Source: three-view drawing plus pictorial views. Frame: mm from the lowest corner of the part. Coordinates: 2 decimals unless noted, no trailing zeros. Write each loop counter-clockwise with the first axis right and the second up, starting at its lowest first coordinate (ties: lowest second). Pieces come first, ordered by that corner, then holes. Notation, with made-up numbers: M -28.75,16 L 15.25,16 A16 cw 15.25,38 Z; hole C 35.5,80 d11. An arc over 180 degrees is marked long. Write item = value, one per line. Start each with the question number.
Item 1: Section A-A on y = 1.2. Output: boundary loops of the cut face in (x, z) (1 decimal).
Item 2: Ray query, L1, parallel to X at y = 1, z = 15.5. Return the intervals inside material, ascending. Write a range as [from, to].
Item 3: Section B-B on z = 36.5. Output: boundary loops of the cut face in (x, y).
Item 4: First-contact query: pin 1 Ø1.6 at (y, z) = (2.5, 42.5) entering from -X; pin 2 Ø3 at (y, z) = (4.5, 78.5) entering from +X; pin 3 Ø1.6 at (x, y) = (4, 3) entering from -Z. Flat tips, straight axial feed; report the tip coordinate or a pass-through.
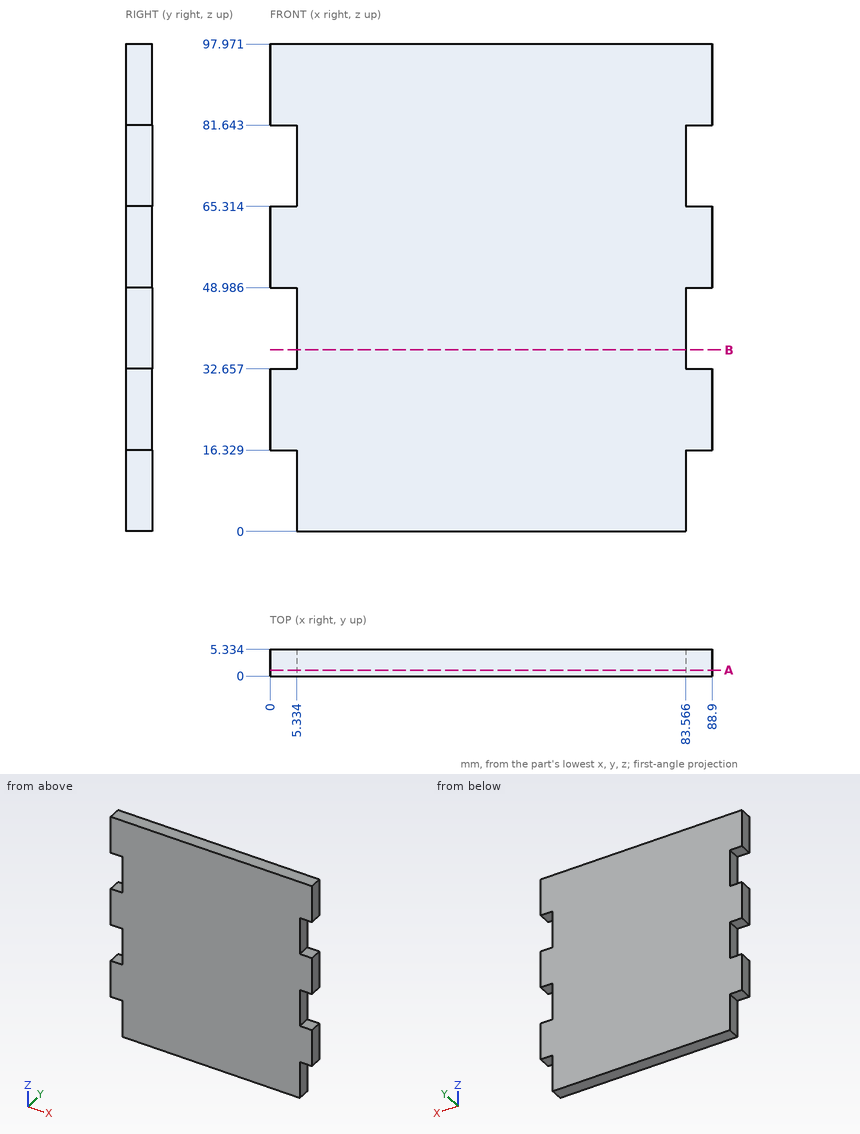
Responses:
q1.outline = M 0,16.3 L 5.3,16.3 L 5.3,0 L 83.6,0 L 83.6,16.3 L 88.9,16.3 L 88.9,32.7 L 83.6,32.7 L 83.6,49 L 88.9,49 L 88.9,65.3 L 83.6,65.3 L 83.6,81.6 L 88.9,81.6 L 88.9,98 L 0,98 L 0,81.6 L 5.3,81.6 L 5.3,65.3 L 0,65.3 L 0,49 L 5.3,49 L 5.3,32.7 L 0,32.7 Z
q2.L1 = [5.33, 83.57]
q3.outline = M 5.33,0 L 83.57,0 L 83.57,5.33 L 5.33,5.33 Z
q4.pin_1 = 5.33
q4.pin_2 = 83.57
q4.pin_3 = 16.33
